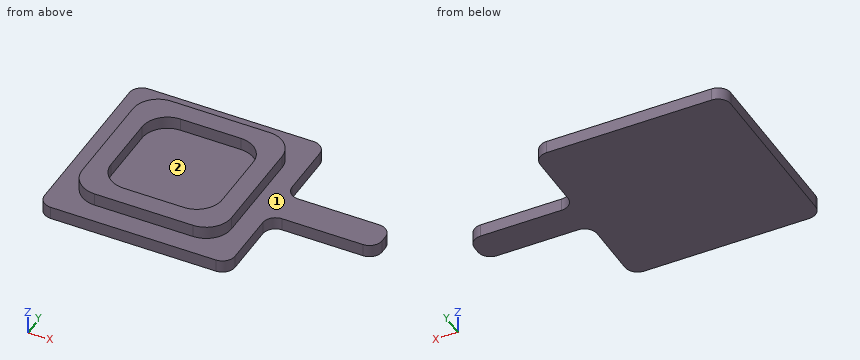
Autodesk Inventor part; units mm, degrees
ref_plane "YZ Plane" through (0, 0, 0) normal (1, 0, 0) x (0, 1, 0)
ref_plane "XZ Plane" through (0, 0, 0) normal (0, 1, 0) x (-1, 0, 0)
ref_plane "XY Plane" through (0, 0, 0) normal (0, 0, 1) x (1, 0, 0)
sketch "Sketch1" plane through (0, 0, 0) normal (0, 0, 1) x (1, 0, 0)
  line L0 (-15, -15) -> (15, -15)
  line L1 (15, -15) -> (15, 15)
  line L2 (15, 15) -> (-15, 15)
  line L3 (-15, 15) -> (-15, -15)
  line L4 (-15, -15) -> (15, 15) construction
  line L5 (15, -15) -> (-15, 15) construction
  line L6 (-11.75, -11.75) -> (11.75, -11.75)
  line L7 (11.75, -11.75) -> (11.75, 11.75)
  line L8 (11.75, 11.75) -> (-11.75, 11.75)
  line L9 (-11.75, 11.75) -> (-11.75, -11.75)
  line L10 (-11.75, -11.75) -> (11.75, 11.75) construction
  line L11 (11.75, -11.75) -> (-11.75, 11.75) construction
  line L12 (-8.75, 8.75) -> (8.75, 8.75)
  line L13 (8.75, 8.75) -> (8.75, -8.75)
  line L14 (8.75, -8.75) -> (-8.75, -8.75)
  line L15 (-8.75, -8.75) -> (-8.75, 8.75)
  line L16 (15, -2.5) -> (31.75, -2.5)
  line L17 (31.75, -2.5) -> (31.75, 2.5)
  line L18 (31.75, 2.5) -> (15, 2.5)
  line L19 (15, 2.5) -> (15, -2.5)
  point P0 (0, 0)
  point P1 (11.75, 0)
  dimension "d0" = 30
  dimension "d1" = 30
  dimension "d2" = 23.5
  dimension "d3" = 23.5
  dimension "d4" = 3
  dimension "d10" = 5
  dimension "d12" = 20
extrude "Extrusion2" add sketch "Sketch1" against normal blind 2 contours L3 L2 L1 L0 | L9 L8 L7 L6 | L12 L13 L14 L15
extrude "Extrusion3" add sketch "Sketch1" against normal blind 2 contours L1 L18 L17 L16
fillet "Fillet2" radius 2 4 edges at (-15, -15, -1) (-15, 15, -1) (15, -15, -1) (15, 15, -1)
fillet "Fillet3" radius 2 4 edges at (31.75, -2.5, -1) (31.75, 2.5, -1) (15, 2.5, -1) (15, -2.5, -1)
extrude "Extrusion4" add sketch "Sketch1" along normal blind 2 contours L9 L8 L7 L6
fillet "Fillet4" radius 4 8 edges at (11.75, 11.75, 1) (11.75, -11.75, 1) (-11.75, -11.75, 1) (-11.75, 11.75, 1) (8.75, 8.75, 1) (-8.75, 8.75, 1) (-8.75, -8.75, 1) (8.75, -8.75, 1)
properties part number "DustCover" material "ABS Plastic"
Here's how the part is built. I have some questions about the finished solid (model axes, mm). Face numbers are marked on the shaded views. Give positions to 0.01 mm unless a question says otherwise; leave off trailing zeros. Write each loop counter-clockwise with the first axis right and the second up, starting at its lowest first coordinate (ties: lowest second). Pieces come first, ordered by that corner, then holes. Notation, with made-up numbers: (6, -8) -> (31, -8) arc R23 cw to (31, 17) -> close; hole circle Ø10 at (4.5, 60.5). An arc over 180 degrees is marked (long way). Write each question's results on one line, items separated by ' | '.
Item 1: Suppose I cut it at C-C on x = -2. Write out the boundary of the cut face in (y, z).
Output:
outline: (-15, -2) -> (15, -2) -> (15, 0) -> (11.75, 0) -> (11.75, 2) -> (8.75, 2) -> (8.75, 0) -> (-8.75, 0) -> (-8.75, 2) -> (-11.75, 2) -> (-11.75, 0) -> (-15, 0) -> close
Item 2: We'd pull the mould along Y, two halves only. Please class the marked faces 1 and 2: pulls with the +Y half, pulls with the -Y half, needs draft (parallel to the pull), parting line crosses it, or undercut.
Output:
face 1: needs draft | face 2: undercut
Item 3: Suppose I cut it at D-D on y = 4. Write out the boundary of the cut face in (x, z).
Output:
outline: (-15, -2) -> (15.06, -2) -> (15.06, 0) -> (11.75, 0) -> (11.75, 2) -> (8.75, 2) -> (8.75, 0) -> (-8.75, 0) -> (-8.75, 2) -> (-11.75, 2) -> (-11.75, 0) -> (-15, 0) -> close
Item 4: For pin 1 Ø0.6 at (y, z) = (1, 1) entering from +X; pin 2 Ø1 at (x, z) = (26, -1) entering from +Y; pin 3 Ø1.5 at (y, z) = (7.5, 1) entering from -X, each with a flat end and sliding along its axis, tell me the tip position at first contact or that it passes through.
Output:
pin 1: stops at x = 11.75 | pin 2: stops at y = 2.5 | pin 3: stops at x = -11.75
Item 5: If I drill on L1, parallel to Y at x = -4, z = 0.7; L2, parallel to Y at x = 5, z = 1.45; L3, parallel to Z at x = 5, y = -12.5, over which ranges is the centre line in solid material (lowest first)?
Output:
L1: y = -11.75 to -8.75, 8.75 to 11.75 | L2: y = -11.75 to -8.74, 8.74 to 11.75 | L3: z = -2 to 0
Item 6: Suppose I cut it at A-A on z = 0.9. Write out the boundary of the cut face in (x, y), plus the area to 3 significant figures.
Output:
outline: (-11.75, -7.75) arc R4 ccw to (-7.75, -11.75) -> (7.75, -11.75) arc R4 ccw to (11.75, -7.75) -> (11.75, 7.75) arc R4 ccw to (7.75, 11.75) -> (-7.75, 11.75) arc R4 ccw to (-11.75, 7.75) -> close; hole (-8.75, -4.75) arc R4 ccw to (-4.75, -8.75) -> (4.75, -8.75) arc R4 ccw to (8.75, -4.75) -> (8.75, 4.75) arc R4 ccw to (4.75, 8.75) -> (-4.75, 8.75) arc R4 ccw to (-8.75, 4.75) -> close | area: 246 mm^2
Item 7: Suppose I cut it at B-B on z = -1.15. Write out the boundary of the cut face in (x, y).
Output:
outline: (-15, -13) arc R2 ccw to (-13, -15) -> (13, -15) arc R2 ccw to (15, -13) -> (15, -4.5) arc R2 cw to (17, -2.5) -> (29.75, -2.5) arc R2 ccw to (31.75, -0.5) -> (31.75, 0.5) arc R2 ccw to (29.75, 2.5) -> (17, 2.5) arc R2 cw to (15, 4.5) -> (15, 13) arc R2 ccw to (13, 15) -> (-13, 15) arc R2 ccw to (-15, 13) -> close
